```python
from build123d import *

# Parameters (mm, degrees)
F1_W     = 1
F1_H     = 3
F1_W_2   = 8
F2_DEPTH = 0.75
F3_DEPTH = 3
F4_R     = 0.75
F5_DEPTH = 10
F6_R     = 1.49999


# Not quite as in the source:
# - a fillet or chamfer is up to 0.001 mm smaller than in the source, because OpenCascade refuses the exact size


with BuildPart() as f2:
    # F1 (on Top) → F2 (new body)
    with BuildSketch(Plane.XY):
        with Locations((4.5, 0)):
            Rectangle(F1_W, F1_H)
        with Locations((-4.5, 0)):
            Rectangle(F1_W, F1_H)
        Rectangle(F1_W_2, F1_H)
    extrude(amount=F2_DEPTH)

    # F1 (on Top) → F3 (join)
    with BuildSketch(Plane.XY):
        with Locations((-4.5, 0)):
            Rectangle(F1_W, F1_H)
        with Locations((4.5, 0)):
            Rectangle(F1_W, F1_H)
    extrude(amount=F3_DEPTH)

    # F4 (on face) → F5 (cut, through all)
    with BuildSketch(Plane(origin=(-5, 0, 0), x_dir=(0, -1, 0), z_dir=(-1, 0, 0))):
        with Locations((0, 1.5)):
            Circle(F4_R)
    extrude(amount=-F5_DEPTH, mode=Mode.SUBTRACT)

    # F6 (radius 1.5 in the source; OpenCascade refuses exactly that, so slightly less here)
    f6_edges = [f2.edges().sort_by_distance(p)[0] for p in [
        (4.5, 1.5, 3),
        (4.5, -1.5, 3),
        (-4.5, -1.5, 3),
        (-4.5, 1.5, 3),
    ]]
    fillet(f6_edges, radius=F6_R)


solid = f2.part
```
Can you work these out from the model? Positions are in its coordinate system, mm. A direction names the side the tool comes from. Coordinates: 2 decimals unless noted, no trailing zeros. Order: outer loops, then holes, each group sorted by start corner. A loop starts at its lowest first (then second) coordinate and runs counter-clockwise, first axis right, second up.
1. For faces 1 (the face through (0.1, 1.5, 0.6)), 2 (the face through (-4, 0.3, 2.4)), which set-ups out of +Z, -Z, +X, -X, +Y, -Y let a thin tool reach every point of the face, with its end or its side?
2. Thinking about a two-plate mould opening in X: for faces 3 (the face through (0, 0, 0)), 4 (the face through (5, -1, 1)), 5 (the face through (0, 0, 0.75)), which applies, +X half, -X half, draft (parallel to the pull), parting line (faces both ways), or undercut?
3. If we section it at A-A (y = 0.6): Please give me the cut outline in (x, z), then the cut area to 3 significant figures.
4. I'm going to push flat-ended pins straight in: pin 1 (1.5 mm diameter, centred on x = 3.5, z = 2.5, fed in from +Y); pin 2 (0.9 mm diameter, centred on x = -1.5, y = -0.5, fed in from +Z). Where does each tip first touch, or does it pass through?
5. If we section it at C-C (x = 2.25): Please give me the cut outline in (y, z), then the cut area to 3 significant figures.
6. If we section it at D-D (y = -1): Please give me the cut outline in (x, z), then the cut area to 3 significant figures.
7. If we section it at B-B (z = 1.15): Please give me the cut outline in (x, y).
8. I need wall thicknesses on line 1 (X direction, y = -0.8, z = 2.4); line 2 (Y direction, x = 4.55, z = 1.5); line 3 (Z direction, x = 4.5, y = 0). Which ranges of each line are inside material? Lowest first, please.
Entries:
1. face 1: +Z, -Z, +X, -X, +Y
1. face 2: +Z, +Y, -Y
2. face 3: draft
2. face 4: +X half
2. face 5: undercut
3. outline: (-5, 0) - (5, 0) - (5, 1.05) - (4, 1.05) - (4, 0.75) - (-4, 0.75) - (-4, 1.05) - (-5, 1.05) - close; (-5, 1.95) - (-4, 1.95) - (-4, 2.87) - (-5, 2.87) - close; (4, 1.95) - (5, 1.95) - (5, 2.87) - (4, 2.87) - close
3. area: 9.95 mm2
4. pin 1: stops at y = 1.43
4. pin 2: stops at z = 0.75
5. outline: (-1.5, 0) - (1.5, 0) - (1.5, 0.75) - (-1.5, 0.75) - close
5. area: 2.25 mm2
6. outline: (-5, 0) - (5, 0) - (5, 2.62) - (4, 2.62) - (4, 0.75) - (-4, 0.75) - (-4, 2.62) - (-5, 2.62) - close
6. area: 11.2 mm2
7. outline: (-5, -1.5) - (-4, -1.5) - (-4, -0.66) - (-5, -0.66) - close; (-5, 0.66) - (-4, 0.66) - (-4, 1.5) - (-5, 1.5) - close; (4, -1.5) - (5, -1.5) - (5, -0.66) - (4, -0.66) - close; (4, 0.66) - (5, 0.66) - (5, 1.5) - (4, 1.5) - close
8. line 1: x = -5 to -4, 4 to 5
8. line 2: y = -1.5 to -0.75, 0.75 to 1.5
8. line 3: z = 0 to 0.75, 2.25 to 3
